```python
from build123d import *

# Parameters (mm, degrees)
F1_DEPTH = 63.5
F2_DEPTH = 25.4
F3_DEPTH = 12.7


with BuildPart() as f1:
    # F0 (on Front) → F1 (new body, symmetric)
    with BuildSketch(Plane.XZ):
        Polygon((41.275, -9.525), (41.275, 9.525), (22.225, 9.525), (-41.275, 9.525), (-41.275, -9.525), align=None)
    extrude(amount=F1_DEPTH, both=True)

    # F0 (on Front) → F2 (join, symmetric)
    with BuildSketch(Plane.XZ):
        with BuildLine():
            Line((22.225, 9.525), (41.275, 9.525))
            Line((41.275, 9.525), (41.275, 27.0002))
            ThreePointArc((41.275, 27.0002), (45.92468, 38.22552), (57.15, 42.8752))
            Line((57.15, 42.8752), (59.910303, 42.8752))
            Line((59.910303, 42.8752), (59.910303, 61.9252))
            Line((59.910303, 61.9252), (57.15, 61.9252))
            ThreePointArc((57.15, 61.9252), (32.454296, 51.695904), (22.225, 27.0002))
            Line((22.225, 27.0002), (22.225, 9.525))
        make_face()
    extrude(amount=F2_DEPTH, both=True)

    # F0 (on Front) → F3 (join, symmetric)
    with BuildSketch(Plane.XZ):
        with BuildLine():
            Line((-41.275, 9.525), (22.225, 9.525))
            Line((22.225, 9.525), (22.225, 27.0002))
            ThreePointArc((22.225, 27.0002), (32.454296, 51.695904), (57.15, 61.9252))
            add(Edge.make_bspline(
                [(-41.275, 9.525), (-41.021902, 37.119821), (13.006945, 62.733494), (57.15, 61.9252)],
                knots=[0, 0, 0, 0, 111.504536, 111.504536, 111.504536, 111.504536], degree=3))
        make_face()
    extrude(amount=F3_DEPTH, both=True)


solid = f1.part
```
Geometry check sheet. Reference: the model listing, model coordinates, mm. A direction names the side the tool comes from. Coordinates: 2 decimals unless noted, no trailing zeros. Order: outer loops, then holes, each group sorted by start corner. A loop starts at its lowest first (then second) coordinate and runs counter-clockwise, first axis right, second up.
Item 1: Depth check by flat-ended pin: pin 1 (1.5 mm diameter, centred on y = -11, z = 17, fed in from -X); pin 2 (2 mm diameter, centred on y = -26.5, z = 27.5, fed in from +X); pin 3 (2 mm diameter, centred on x = -30.5, y = 31.5, fed in from +Z) (3 decimals); pin 4 (11 mm diameter, centred on y = 29, z = 10.5, fed in from +X) (3 decimals). Enter the tip coordinate at first touch or a pass-through.
Item 2: Scan lines: line 1 along Y through (x, z) = (-34.5, 10); line 2 along Z through (x, y) = (-8, -35) (3 decimals); line 3 along X through (y, z) = (-13.5, 18) (3 decimals). Record each from-to range of solid material in increasing order.
Item 3: Tool access check on faces 1 (the flat face through (37, -25.4, 36)), 2 (the cylindrical face through (32.73, 18.96, 51.97)), 3 (the flat face through (22.225, -19, 18)), 4 (the flat face through (41.275, -1, 4)). Record the directions out of +Z, -Z, +X, -X, +Y, -Y that give a thin tool (end or side, any length) a straight path to the whole face; none if there is none.
Item 4: Section check A-A (y = 16). Enter the section's corners in (x, z) (3 decimals).
Item 5: Section check C-C (y = 49.5). Enter the section's corners in (x, z) (3 decimals).
Item 6: Section check B-B (z = 6). Enter the section's corners in (x, y) (3 decimals).
Check sheet entries:
1. pin 1: stops at x = -40.17
1. pin 2: passes through
1. pin 3: stops at z = 9.525
1. pin 4: stops at x = 41.275
2. line 1: y = -12.7 to 12.7
2. line 2: z = -9.525 to 9.525
2. line 3: x = 22.225 to 41.275
3. face 1: +Z, +X, -X, -Y
3. face 2: +Z, -X, +Y
3. face 3: +Z, -X, -Y
3. face 4: -Z, +X, +Y, -Y
4. outline: (-41.275, -9.525) - (41.275, -9.525) - (41.275, 27) arc R15.875 cw to (57.15, 42.875) - (59.91, 42.875) - (59.91, 61.925) - (57.15, 61.925) arc R34.925 ccw to (22.225, 27) - (22.225, 9.525) - (-41.275, 9.525) - close
5. outline: (-41.275, -9.525) - (41.275, -9.525) - (41.275, 9.525) - (-41.275, 9.525) - close
6. outline: (-41.275, -63.5) - (41.275, -63.5) - (41.275, 63.5) - (-41.275, 63.5) - close
